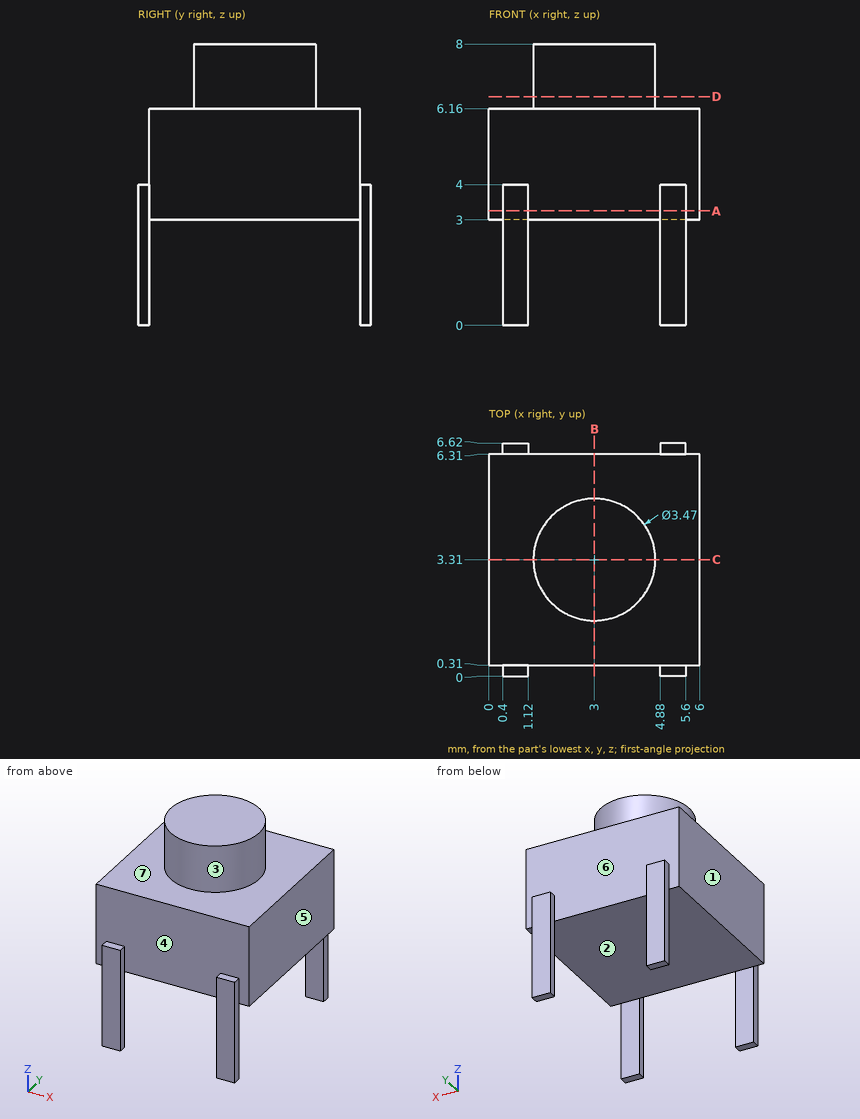
Could you check a few things on this drawing? It's one solid part, dimensions in mm from its lowest x, y, z. A direction names the side the tool comes from. Round coordinates to 2 decimals unless told otherwise and drop trailing zeros. Loops run counter-clockwise (first coordinate to the right, second up) from the corner with the lowest first, then second, coordinate; pieces in that order, holes last. Notation, with made-up numbers: (-19.75, 19) -> (-14.75, 19) arc R13 ccw to (-14.75, 25) -> close; hole circle Ø11 at (46.25, 46.5). An arc over 180 degrees is marked (long way). Answer as CSV lines item,"result".
1. If we section it at B-B on x = 3: Please give me the cut outline in (y, z) (3 decimals), plus the area to 3 significant figures.
Final values:
outline,"(0.31, 3) -> (6.31, 3) -> (6.31, 6.16) -> (5.045, 6.16) -> (5.045, 8) -> (1.575, 8) -> (1.575, 6.16) -> (0.31, 6.16) -> close"
area,"25.3 mm^2"
2. For pin 1 (2.5 mm diameter, centred on x = 3, z = 4.5, fed in from -Y); pin 2 (3.5 mm diameter, centred on x = 3, z = 5, fed in from +Y); pin 3 (1.5 mm diameter, centred on x = 2, y = 1.5, fed in from -Z), each with a flat end and sliding along its axis, tell me the tip position at first contact or that it passes through.
Final values:
pin 1,"stops at y = 0.31"
pin 2,"stops at y = 6.31"
pin 3,"stops at z = 3"
3. If we section it at D-D on z = 6.5: Please give me the cut outline in (x, y) (3 decimals), plus the area to 3 significant figures.
Final values:
outline,"circle Ø3.47 at (3, 3.31)"
area,"9.46 mm^2"
4. If we section it at C-C on y = 3.31: Please give me the cut outline in (x, z) (3 decimals), plus the area to 3 significant figures.
Final values:
outline,"(0, 3) -> (6, 3) -> (6, 6.16) -> (4.735, 6.16) -> (4.735, 8) -> (1.265, 8) -> (1.265, 6.16) -> (0, 6.16) -> close"
area,"25.3 mm^2"
5. Thinking about a two-plate mould opening in X: for the marked faces 4, 5, 6 and 7, which applies, released by +X, released by -X, zero draft, split by the parting line, or undercut?
Final values:
face 4,"undercut"
face 5,"released by +X"
face 6,"undercut"
face 7,"zero draft"
6. If we section it at A-A on z = 3.25: Please give me the cut outline in (x, y).
Final values:
outline,"(0, 0.31) -> (0.4, 0.31) -> (0.4, 0) -> (1.12, 0) -> (1.12, 0.31) -> (4.88, 0.31) -> (4.88, 0) -> (5.6, 0) -> (5.6, 0.31) -> (6, 0.31) -> (6, 6.31) -> (5.6, 6.31) -> (5.6, 6.62) -> (4.88, 6.62) -> (4.88, 6.31) -> (1.12, 6.31) -> (1.12, 6.62) -> (0.4, 6.62) -> (0.4, 6.31) -> (0, 6.31) -> close"
7. If I drill on L1, parallel to Z at x = 1.25, y = 3; L2, parallel to Z at x = 4.4, y = 3; L3, parallel to Y at x = 3.35, z = 4.75, over which ranges is the centre line in solid material (lowest first)?
Final values:
L1,"z = 3 to 6.16"
L2,"z = 3 to 8"
L3,"y = 0.31 to 6.31"
8. Which directions (+Z, -Z, +X, -X, +Y, -Y) give clear straight access to the entire face, cutting with the end or side of a thin tool? Please do the marked faces 1, 2 and 3.
Final values:
face 1,"+Z, -Z, -X, +Y, -Y"
face 2,"-Z, +X, -X"
face 3,"+Z"
